The listing builds one solid part. Answer for the finished solid, in the listing's coordinates (mm). Face numbers are marked on the shaded views. A direction names the side the tool comes from. Round coordinates to 2 decimals unless told otherwise and drop trailing zeros. Write each loop counter-clockwise with the first axis right and the second up, starting at its lowest first coordinate (ties: lowest second). Pieces come first, ordered by that corner, then holes. Notation, with made-up numbers: (25, 32.5) - (30, 32.5) arc R24 ccw to (30, 67.5) - close; hole circle Ø10 at (-31, 10). An arc over 180 degrees is marked (long way). Answer in a Markdown table with one row per item.
from build123d import *

# Parameters (mm, degrees)
SKETCH1_R               = 7.5
BOSS_EXTRUDE1_DEPTH     = 8.5
CUT_EXTRUDE1_DEPTH      = 6.8
SKETCH3_R               = 1.5
CUT_EXTRUDE2_DEPTH      = 11.2
CUT_EXTRUDE2_DEPTH_BACK = 5.8
FILLET1_R               = 1.5


with BuildPart() as part:
    # Sketch1 → Boss-Extrude1 (new body)
    with BuildSketch(Plane.XY):
        Circle(SKETCH1_R)
    extrude(amount=BOSS_EXTRUDE1_DEPTH)

    # Sketch2 → Cut-Extrude1 (cut)
    with BuildSketch(Plane.XY.offset(8.5)):
        Polygon((2.7, 0), (2.7, 13.78279584), (-2.7, 13.78279584), (-2.7, 0), (-2.7, -14.12853377), (2.7, -14.12853377), align=None)
    extrude(amount=-CUT_EXTRUDE1_DEPTH, mode=Mode.SUBTRACT)

    # Sketch3 → Cut-Extrude2 (cut, two sides)
    with BuildSketch(Plane(origin=(-2.7, 0, 0), x_dir=(0, 0, -1), z_dir=(1, 0, 0))) as cut_extrude2_sk:
        with Locations((-5.3, 0)):
            Circle(SKETCH3_R)
    extrude(amount=CUT_EXTRUDE2_DEPTH, mode=Mode.SUBTRACT)
    extrude(cut_extrude2_sk.sketch, amount=-CUT_EXTRUDE2_DEPTH_BACK, mode=Mode.SUBTRACT)

    # Fillet1
    fillet1_edges = [part.edges().sort_by_distance(p)[0] for p in [
        (-2.7, 0, 1.7),
        (2.7, 0, 1.7),
        (2.7, 0, 8.5),
        (-2.7, 0, 8.5),
    ]]
    fillet(fillet1_edges, radius=FILLET1_R)


solid = part.part
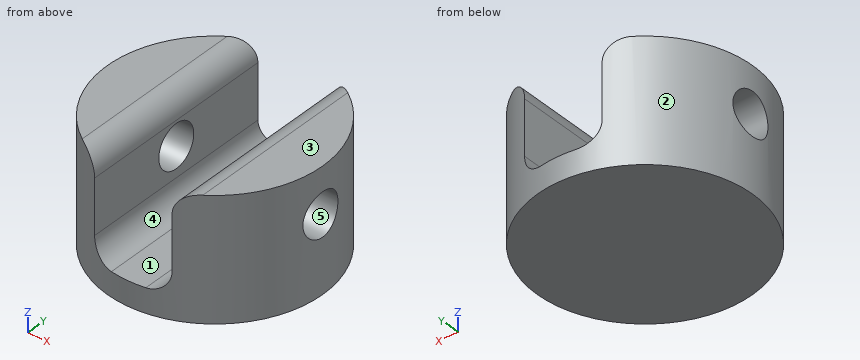
(1) Section D-D (z = 3.5) is taken. Give the vertices of the cut face in (x, y), and give its area (3 significant figures).
Checked values:
| item | result |
|---|---|
| outline | (-2.7, -7) - (-2.7, 7) arc R7.5 ccw to start; (2.7, -7) arc R7.5 ccw to (2.7, 7) - close |
| area | 97.5 mm2 |
(2) Section C-C (x = -5.5) is taken. Give the vertices of the cut face in (y, z), and give its area (3 significant figures).
Checked values:
| item | result |
|---|---|
| outline | (-5.1, 0) - (5.1, 0) - (5.1, 8.5) - (-5.1, 8.5) - close; hole circle Ø3 at (0, 5.3) |
| area | 79.6 mm2 |
(3) Section A-A (z = 6.25) is taken. Give the vertices of the cut face in (x, y).
Checked values:
| item | result |
|---|---|
| outline | (-7.41, -1.16) arc R7.5 ccw to (-2.7, -7) - (-2.7, -1.16) - close; (-7.41, 1.16) - (-2.7, 1.16) - (-2.7, 7) arc R7.5 ccw to start; (2.7, -7) arc R7.5 ccw to (7.41, -1.16) - (2.7, -1.16) - close; (2.7, 1.16) - (7.41, 1.16) arc R7.5 ccw to (2.7, 7) - close |
(4) Flat-ended cylindrical pins translate along their axes: pin 1 (1.8 mm diameter, centred on y = 0, z = 5.3, fed in from +X); pin 2 (5 mm diameter, centred on x = -5.5, z = 7.5, fed in from +Y); pin 3 (0.7 mm diameter, centred on x = -0.5, y = 1.5, fed in from +Z); pin 4 (3 mm diameter, centred on x = 1, y = -2, fed in from +Z). Find the tip coordinate at first contact, or state that the pin passes through.
Checked values:
| item | result |
|---|---|
| pin 1 | passes through |
| pin 2 | stops at y = 6.87 |
| pin 3 | stops at z = 1.7 |
| pin 4 | stops at z = 2.45 |
(5) For the marked faces 4 and 5, determine the directions among +Z, -Z, +X, -X, +Y, -Y from which every point of the face is accessible in a straight line to the end or side of a thin tool.
Checked values:
| item | result |
|---|---|
| face 4 | +Z, +Y, -Y |
| face 5 | +X, -X |
(6) For a pull along X with two mould halves and no side action, classify the marked faces 1, 2 and 3 as pulls with the +X half, pulls with the -X half, needs draft (parallel to the pull), parting line crosses it, or undercut.
Checked values:
| item | result |
|---|---|
| face 1 | undercut |
| face 2 | parting line crosses it |
| face 3 | needs draft |
(7) Find the intervals of material crossed by line 1 (Z direction, x = -5.7, y = 0); line 2 (X direction, y = 5, z = 4); line 3 (Y direction, x = -3.75, z = 5.3), in increasing order.
Checked values:
| item | result |
|---|---|
| line 1 | z = 0 to 3.8, 6.8 to 8.5 |
| line 2 | x = -5.59 to -2.7, 2.7 to 5.59 |
| line 3 | y = -6.5 to -1.5, 1.5 to 6.5 |
(8) Section B-B (y = 0) is taken. Give the vertices of the cut face in (x, z), and give its area (3 significant figures).
Checked values:
| item | result |
|---|---|
| outline | (-7.5, 0) - (7.5, 0) - (7.5, 3.8) - (2.7, 3.8) - (2.7, 3.2) arc R1.5 cw to (1.2, 1.7) - (-1.2, 1.7) arc R1.5 cw to (-2.7, 3.2) - (-2.7, 3.8) - (-7.5, 3.8) - close; (-7.5, 6.8) - (-2.7, 6.8) - (-2.7, 7) arc R1.5 ccw to (-4.2, 8.5) - (-7.5, 8.5) - close; (2.7, 6.8) - (7.5, 6.8) - (7.5, 8.5) - (4.2, 8.5) arc R1.5 ccw to (2.7, 7) - close |
| area | 62.0 mm2 |
